Could you check a few things on this model? Use its own coordinates, in mm. Give positions to 0.01 mm unless a question says otherwise; leave off trailing zeros. Order: outer loops, then holes, each group sorted by start corner. A loop starts at its lowest first (then second) coordinate and runs counter-clockwise, first axis right, second up. Notation, with made-up numbers: (22, -11.5) -> (67, -11.5) arc R32 cw to (67, 14.5) -> close; hole circle Ø6 at (38, 33). An arc over 180 degrees is marked (long way). Answer as CSV lines item,"result". Start each with the question number.
(1) I need wall thicknesses on L1, parallel to X at y = 1.85, z = 0; L2, parallel to X at y = 0.55, z = -159; L3, parallel to Z at x = 20.5, y = 0.7. Which ranges of each line are inside material? Lowest first, please.
(2) I want a section at B-B (x = -40). Please give me the cut outline in (y, z), plus the area to 3 significant figures.
(3) Will these pins go through, and if not, where does the flat tip stop? pin 1 Ø1.5 at (x, y) = (51, 1.5) entering from +Z; pin 2 Ø1 at (x, y) = (18, 1.5) entering from -Z.
(4) I want a section at C-C (y = 1.95). Give the number of separate pieces and of enclosed holes in the cut face, plus the area to 3 significant figures.
(5) I want a section at D-D (z = -118). Please give me the cut outline in (x, y).
(6) We'd pull the mould along X, two halves only. Please class faces 1 (the face through (99.487, 1.479, -79.882)), 2 (the face through (-28.35, 1.52, 28.22)), 3 (the face through (26, 3, -37)): released by +X, released by -X, zero draft, split by the parting line, or undercut.
(7) I want a section at A-A (x = 0). Please give me the cut outline in (y, z).
```python
from build123d import *

# Parameters (mm, degrees)
IZIM1_R               = 50
TOP_COVER_DEPTH       = 3
IZIM2_R               = 2
SPACER_DELIKLER_DEPTH = 71.774289117
IZIM4_R               = 5
KES_EKSTR_ZYON3_DEPTH = 71.774289117
IZIM4_3_R             = 1.5
KES_EKSTR_ZYON4_DEPTH = 71.774289117
KANCA_START           = -3
KANCA_DELIKLERI_DEPTH = 3


with BuildPart() as part:
    # izim1 → top cover (new body)
    with BuildSketch(Plane(origin=(0, 0, 0), x_dir=(1, 0, 0), z_dir=(0, 1, 0))):
        with Locations(Location((0, 0, 0), (0, 0, 270))):
            Circle(IZIM1_R)
    extrude(amount=TOP_COVER_DEPTH)

    # izim2 → spacer delikler (cut, through all)
    with BuildSketch(Plane(origin=(0, 3, 0), x_dir=(1, 0, 0), z_dir=(0, 1, 0))):
        with Locations(Location((-29.69848481, 29.69848481, 0), (0, 0, 270))):
            Circle(IZIM2_R)
        with Locations(Location((29.69848481, 29.69848481, 0), (0, 0, 270))):
            Circle(IZIM2_R)
        with Locations(Location((29.69848481, -29.69848481, 0), (0, 0, 270))):
            Circle(IZIM2_R)
        with Locations(Location((-29.69848481, -29.69848481, 0), (0, 0, 270))):
            Circle(IZIM2_R)
    extrude(amount=-SPACER_DELIKLER_DEPTH, mode=Mode.SUBTRACT)

    # izim4 → Kes-Ekstr_zyon3 (cut, through all)
    with BuildSketch(Plane(origin=(0, 3, 0), x_dir=(1, 0, 0), z_dir=(0, 1, 0))):
        with Locations(Location((0, 0, 0), (0, 0, 270))):
            Circle(IZIM4_R)
    extrude(amount=-KES_EKSTR_ZYON3_DEPTH, mode=Mode.SUBTRACT)

    # izim4_3 → Kes-Ekstr_zyon4 (cut, through all)
    with BuildSketch(Plane(origin=(0, 3, 0), x_dir=(1, 0, 0), z_dir=(0, 1, 0))):
        with Locations(Location((34.079267821, 12.675680455, 0), (0, 0, 270))):
            Circle(IZIM4_3_R)
        with Locations(Location((32.362523879, -1.361868841, 0), (0, 0, 270))):
            Circle(IZIM4_3_R)
        with Locations(Location((18.324974583, 0.354875101, 0), (0, 0, 270))):
            Circle(IZIM4_3_R)
        with Locations(Location((20.041718525, 14.392424397, 0), (0, 0, 270))):
            Circle(IZIM4_3_R)
    extrude(amount=-KES_EKSTR_ZYON4_DEPTH, mode=Mode.SUBTRACT)

    # izim3 → kanca delikleri (add)
    with BuildSketch(Plane(origin=(0, 3, 0), x_dir=(1, 0, 0), z_dir=(0, 1, 0)).offset(KANCA_START)):
        with BuildLine():
            ThreePointArc((48.06829925, 13.763669832), (49.2554017, 8.596825189), (49.888765157, 3.333333333))
            ThreePointArc((49.888765157, 3.333333333), (99.613854084, 81.220474128), (64.278760969, 166.604444312))
            ThreePointArc((64.278760969, 166.604444312), (50.190440441, 165.371875978), (51.423008775, 151.28355545))
            ThreePointArc((51.423008775, 151.28355545), (69.056591634, 86.88644621), (15, 47.696960071))
            ThreePointArc((15, 47.696960071), (35.531564272, 35.178231058), (47.844482908, 14.522584318))
            ThreePointArc((47.844482908, 14.522584318), (48.609720304, 15.376680878), (49.674237351, 14.950215566))
            ThreePointArc((49.674237351, 14.950215566), (49.795665804, 14.688455458), (49.837297416, 14.402920816))
            ThreePointArc((49.837297416, 14.402920816), (49.177151674, 13.462442702), (48.06829925, 13.763669832))
        make_face()
        with BuildLine():
            ThreePointArc((66.018615213, 27.769945559), (65.40884087, 26.849226309), (64.32316734, 27.051369011))
            ThreePointArc((64.32316734, 27.051369011), (64.296186155, 28.461390608), (65.706036097, 28.496204829))
            ThreePointArc((65.706036097, 28.496204829), (65.937152334, 28.1652803), (66.018615213, 27.769945559))
        make_face(mode=Mode.SUBTRACT)
        with BuildLine():
            ThreePointArc((78.663944618, 44.521304918), (78.158866275, 43.652367317), (77.153839511, 43.661192844))
            ThreePointArc((77.153839511, 43.661192844), (76.8010119, 45.026623752), (78.164461583, 45.387031646))
            ThreePointArc((78.164461583, 45.387031646), (78.530119244, 45.021046368), (78.663944618, 44.521304918))
        make_face(mode=Mode.SUBTRACT)
        with BuildLine():
            ThreePointArc((87.08557892, 63.745988838), (86.678444563, 62.940687448), (85.788558261, 62.791117785))
            ThreePointArc((85.788558261, 62.791117785), (85.129072487, 64.037700073), (86.371971728, 64.704101127))
            ThreePointArc((86.371971728, 64.704101127), (86.887574184, 64.343319229), (87.08557892, 63.745988838))
        make_face(mode=Mode.SUBTRACT)
        with BuildLine():
            ThreePointArc((90.825513882, 84.398477371), (90.508235288, 83.667798589), (89.757730918, 83.400777281))
            ThreePointArc((89.757730918, 83.400777281), (88.827452617, 84.460716511), (89.882207277, 85.396869007))
            ThreePointArc((89.882207277, 85.396869007), (90.552388492, 85.085247567), (90.825513882, 84.398477371))
        make_face(mode=Mode.SUBTRACT)
        with BuildLine():
            ThreePointArc((89.680355962, 105.355600491), (89.443619041, 104.70951267), (88.845497016, 104.369330532))
            ThreePointArc((88.845497016, 104.369330532), (87.695018674, 105.184982708), (88.504266716, 106.339974697))
            ThreePointArc((88.504266716, 106.339974697), (89.322193462, 106.122441168), (89.680355962, 105.355600491))
        make_face(mode=Mode.SUBTRACT)
        with BuildLine():
            ThreePointArc((58.850884872, 158.943999881), (58.789623808, 158.59937079), (58.613346451, 158.296966388))
            ThreePointArc((58.613346451, 158.296966388), (56.912145936, 159.288628972), (58.850884872, 158.943999881))
        make_face(mode=Mode.SUBTRACT)
        with BuildLine():
            ThreePointArc((83.712383709, 125.47762085), (83.545775574, 124.924938302), (83.10146771, 124.556418571))
            ThreePointArc((83.10146771, 124.556418571), (81.793357223, 125.083425063), (82.313088302, 126.394443177))
            ThreePointArc((82.313088302, 126.394443177), (83.260427773, 126.314070313), (83.712383709, 125.47762085))
        make_face(mode=Mode.SUBTRACT)
        with BuildLine():
            ThreePointArc((73.246160797, 143.670217534), (73.138311823, 143.218480281), (72.838027705, 142.864181825))
            ThreePointArc((72.838027705, 142.864181825), (71.443425677, 143.073881783), (71.64537461, 144.469627289))
            ThreePointArc((71.64537461, 144.469627289), (72.692934684, 144.564864444), (73.246160797, 143.670217534))
        make_face(mode=Mode.SUBTRACT)
    extrude(amount=KANCA_DELIKLERI_DEPTH)


solid = part.part
```
Final values:
1,L1,"-50 to -5, 5 to 16.87, 19.78 to 31.73, 32.99 to 50"
1,L2,"47.85 to 56.85, 58.85 to 72.38"
1,L3,"-48.08 to -15.82, -12.96 to 45.6"
2,outline,"(0, -30) -> (3, -30) -> (3, 30) -> (0, 30) -> close"
2,area,"180 mm²"
3,pin 1,"z = -3.54"
3,pin 2,"z = -47.88"
4,separate pieces,"1"
4,enclosed holes,"18"
4,area,"12,900 mm²"
5,outline,"(71.21, 0) -> (96, 0) -> (96, 3) -> (71.21, 3) -> close"
6,face 1,"released by +X"
6,face 2,"undercut"
6,face 3,"zero draft"
7,outline,"(0, -50) -> (3, -50) -> (3, -5) -> (0, -5) -> close; (0, 5) -> (3, 5) -> (3, 50) -> (0, 50) -> close"
